Autodesk Fusion 360 part; units mm, degrees
sketch "Sketch1" plane through (0, 0, 0) normal (0, 0, 1) x (1, 0, 0) in component "BrickHolder"
  line L0 (0, 0) -> (-110, 0)
  line L1 (-110, 0) -> (-110, 51)
  line L2 (-110, 51) -> (0, 51)
  line L3 (0, 51) -> (0, 0)
  dimension "d1" = 110
  dimension "d2" = 51
extrude "Extrude1" add sketch "Sketch1" along normal blind 95 in component "BrickHolder"
sketch "Sketch2" plane through (-110, 0, 0) normal (-1, 0, 0) x (0, -1, 0) in component "BrickHolder"
  line L0 (-51, 0) -> (0, 0)
  line L1 (0, 0) -> (0, 95)
  line L2 (0, 95) -> (-51, 95)
  line L3 (-51, 95) -> (-51, 0)
  line L4 (0, 95) -> (-47, 95)
  line L5 (-47, 95) -> (-47, 35)
  line L6 (-47, 35) -> (0, 35)
  line L7 (0, 35) -> (0, 95)
  dimension "d5" = 47
  dimension "d6" = 60
extrude "Extrude2" cut sketch "Sketch2" against normal blind 140 contours L1 L2 L4 L5 L6 L7 in component "BrickHolder"
sketch "Sketch3" plane through (0, 0, 35) normal (0, 0, 1) x (-1, 0, 0) in component "BrickHolder"
  line L0 (0, 0) -> (0, -47)
  line L1 (0, -47) -> (110, -47)
  line L2 (110, -47) -> (110, 0)
  line L3 (110, 0) -> (0, 0)
  line L4 (0, -47) -> (3.5, -47) construction
  line L5 (110, -47) -> (106.5, -47) construction
  line L6 (0, 0) -> (3.5, 0) construction
  line L7 (3.5, 0) -> (3.5, -3.5) construction
  line L8 (3.5, -3.5) -> (0, -3.5) construction
  line L9 (0, -3.5) -> (0, 0) construction
  line L10 (110, 0) -> (106.5, 0) construction
  line L11 (106.5, 0) -> (106.5, -3.5) construction
  line L12 (106.5, -3.5) -> (110, -3.5) construction
  line L13 (110, -3.5) -> (110, 0) construction
  line L14 (106.5, -47) -> (3.5, -47)
  line L15 (3.5, -47) -> (3.5, -3.5)
  line L16 (3.5, -3.5) -> (106.5, -3.5)
  line L17 (106.5, -3.5) -> (106.5, -47)
  dimension "d9" = 3.5
  dimension "d10" = 3.5
  dimension "d11" = 3.5
  dimension "d12" = 3.5
  dimension "d13" = 3.5
  dimension "d14" = 3.5
extrude "Extrude3" cut sketch "Sketch3" against normal blind 32 contours L1 L14 L15 L16 L17 in component "BrickHolder"
sketch "Sketch4" plane through (0, 0, 0) normal (0, -1, 0) x (1, 0, 0) in component "BrickHolder"
  line L0 (0, 35) -> (-110, 35)
  line L1 (-110, 35) -> (-110, 0)
  line L2 (-110, 0) -> (0, 0)
  line L3 (0, 0) -> (0, 35)
  line L4 (0, 0) -> (-30, 0) construction
  line L5 (-110, 35) -> (-90, 35) construction
  line L6 (0, 35) -> (-20, 35) construction
  line L7 (-110, 0) -> (-80, 0) construction
  line L8 (-90, 35) -> (-80, 0)
  line L9 (-30, 0) -> (-20, 35)
  line L10 (-20, 35) -> (-90, 35)
  line L11 (-80, 0) -> (-30, 0)
  dimension "d17" = 30
  dimension "d18" = 20
  dimension "d19" = 20
  dimension "d20" = 30
extrude "Extrude4" cut sketch "Sketch4" against normal blind 40 contours L0 L2 L8 L9 L10 L11 in component "BrickHolder"
sketch "Sketch5" plane through (0, 47, 0) normal (0, -1, 0) x (1, 0, 0) in component "BrickHolder"
  line L0 (0, 35) -> (0, 95)
  line L1 (0, 95) -> (-110, 95)
  line L2 (-110, 95) -> (-110, 35)
  line L3 (-110, 35) -> (-106.5, 35)
  line L4 (-106.5, 35) -> (-106.5, 3)
  line L5 (-106.5, 3) -> (-3.5, 3)
  line L6 (-3.5, 3) -> (-3.5, 35)
  line L7 (-3.5, 35) -> (0, 35)
  line L8 (-110, 95) -> (-95, 95) construction
  line L9 (-95, 95) -> (-95, 80) construction
  line L10 (-95, 80) -> (-110, 80) construction
  line L11 (-110, 80) -> (-110, 95) construction
  line L12 (0, 95) -> (-15, 95) construction
  line L13 (-15, 95) -> (-15, 80) construction
  line L14 (-15, 80) -> (0, 80) construction
  line L15 (0, 80) -> (0, 95) construction
  circle A0 centre (-95, 80) radius 2.125
  circle A1 centre (-15, 80) radius 2.125
  dimension "d23" = 15
  dimension "d24" = 15
  dimension "d25" = 15
  dimension "d26" = 15
  dimension "d27" = 4.25
  dimension "d28" = 4.25
extrude "Extrude5" cut sketch "Sketch5" against normal blind 45 contours A0 | A1 in component "BrickHolder"
chamfer "Chamfer1" distance 2 angle 45 2 edges at (-96.9812, 47, 80.7684) (-16.9812, 47, 80.7684) in component "BrickHolder"
move_face "OffsetFaces1" offset 15 1 faces at (-1.1667, 16.8333, 35) in component "BrickHolder"
move_face "OffsetFaces2" offset 15 1 faces at (-108.8333, 16.8333, 35) in component "BrickHolder"
move_face "OffsetFaces3" offset -0.5 1 faces at (-67.8917, 51, 26.1129) in component "BrickHolder"
component "BrickHolder" placed x (1, 0, 0) y (0, 1, 0) z (0, 0, 1) at (0, 0, 0)
Design review of the part built by this model. Coordinates are the model's own, in mm. A direction names the side the tool comes from. Round coordinates to 2 decimals unless told otherwise and drop trailing zeros. Write each loop counter-clockwise with the first axis right and the second up, starting at its lowest first coordinate (ties: lowest second). Pieces come first, ordered by that corner, then holes.
Item 1: For faces 1 (the flat face through (-54, 44, 3)), 2 (the flat face through (-26, 2, 14)), 3 (the flat face through (-3, 20, 50)), 4 (the conical face through (-15.293, 48.875, 82.231)), list the 3-axis set-ups (+Z, -Z, +X, -X, +Y, -Y) from which the entire face can be reached by the end or side of a thin tool; tool diameter is ignored.
Item 2: Consider section D-D on z = 35. Give the boundary of the cut face in (x, y).
Item 3: Consider section C-C on x = -33.5. Give the boundary of the cut face in (y, z), and give its area (4 significant figures).
Item 4: For pin 1 Ø12.5 at (x, y) = (-7.5, 25.5) entering from +Z; pin 2 Ø0.9 at (x, z) = (-55.5, 2) entering from -Y; pin 3 Ø8 at (y, z) = (6, 31) entering from +X; pin 4 Ø4.5 at (x, y) = (-102, 23) entering from +Z, all flat-tipped, find the tip position at first contact; note any pin that passes through.
Item 5: Wall thickness on L1, parallel to X at y = 49.55, z = 80 (3 decimals); L2, parallel to X at y = 8, z = 9.5; L3, parallel to Z at x = -15, y = 50.1 (3 decimals): over which ranges is each line inside the solid? List them lowest first.
Item 6: Draft analysis for pull direction X (two halves, no side actions). For faces 5 (the flat face through (-56, 50.5, 47)), 6 (the flat face through (-106.5, 25, 27)), 7 (the flat face through (-13, 3.5, 27)), state which applies: released by +X, released by -X, zero draft, split by the parting line, or undercut.
Item 7: Consider section B-B on y = 25. Give the boundary of the cut face in (x, z), and give its area (3 significant figures).
Item 8: Consider section A-A on z = 80. Give the boundary of the cut face in (x, y) (3 decimals), and give its area (3 significant figures).
Check values:
1. face 1: +Z
1. face 2: +Z, -Y
1. face 3: +Z, +X, -X, -Y
1. face 4: -Y
2. outline: (-110, 0) - (-90, 0) - (-90, 3.5) - (-106.5, 3.5) - (-106.5, 47) - (-3.5, 47) - (-3.5, 3.5) - (-20, 3.5) - (-20, 0) - (0, 0) - (0, 50.5) - (-110, 50.5) - close
3. outline: (40, 0) - (50.5, 0) - (50.5, 95) - (47, 95) - (47, 3) - (40, 3) - close
3. area: 353.5 mm2
4. pin 1: stops at z = 50
4. pin 2: stops at y = 40
4. pin 3: stops at x = 0
4. pin 4: stops at z = 3
5. L1: x = -110 to -97.125, -92.875 to -17.125, -12.875 to 0
5. L2: x = -110 to -106.5, -3.5 to 0
5. L3: z = 0 to 77.875, 82.125 to 95
6. face 5: zero draft
6. face 6: undercut
6. face 7: undercut
7. outline: (-110, 0) - (-80, 0) - (-80.86, 3) - (-106.5, 3) - (-106.5, 50) - (-110, 50) - close; (-30, 0) - (0, 0) - (0, 50) - (-3.5, 50) - (-3.5, 3) - (-29.14, 3) - close
7. area: 506 mm2
8. outline: (-110, 47) - (-99.125, 47) - (-97.125, 49) - (-97.125, 50.5) - (-110, 50.5) - close; (-92.875, 49) - (-90.875, 47) - (-19.125, 47) - (-17.125, 49) - (-17.125, 50.5) - (-92.875, 50.5) - close; (-12.875, 49) - (-10.875, 47) - (0, 47) - (0, 50.5) - (-12.875, 50.5) - close
8. area: 347 mm2
